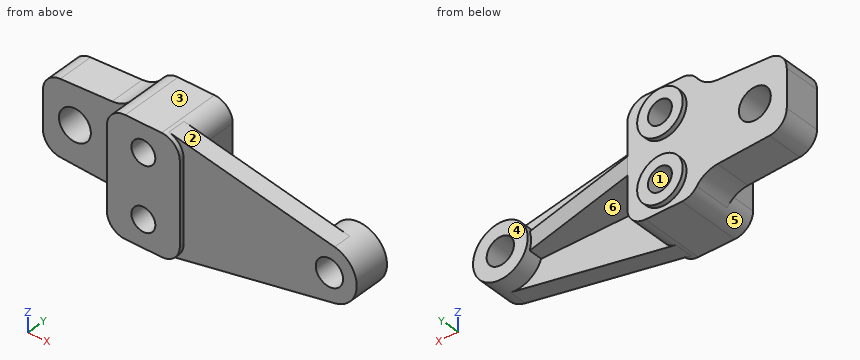
from build123d import *

# Parameters (mm, degrees)
SKETCH1_R                = 8.334375
SKETCH1_R_2              = 19.05
SKETCH1_R_3              = 9.525
SKETCH1_R_4              = 15.875
BOSS_EXTRUDE3_DEPTH      = 12.7
BOSS_EXTRUDE4_DEPTH      = 41.275
BOSS_EXTRUDE4_DEPTH_BACK = 3.175
SKETCH1_5_R              = 8.334375
SKETCH1_5_R_2            = 15.875
SKETCH1_6_R              = 19.05
SKETCH1_6_R_2            = 9.525
BOSS_EXTRUDE5_DEPTH      = 25.4
RIB1_START               = -6.35
RIB1_DEPTH               = 12.7
BOSS_EXTRUDE6_START      = 41.275
SKETCH1_7_R              = 15.875
SKETCH1_7_R_2            = 8.334375
BOSS_EXTRUDE6_DEPTH      = 3.175
BOSS_EXTRUDE8_START      = -25.4
SKETCH4_R                = 11.1125
BOSS_EXTRUDE8_DEPTH      = 25.4


# Read off the part's stored shape, not the designer's step: Rib1
with BuildPart() as part:
    # Sketch1 → Boss-Extrude3 (new body)
    # profile 1 of 5: a face of its own
    with BuildSketch(Plane(origin=(0, 0, 0), x_dir=(1, 0, 0), z_dir=(0, 1, 0))):
        with BuildLine():
            ThreePointArc((40.51167311, 41.043914661), (47.895872817, 36.657751744), (50.8, 28.575))
            Line((50.8, 28.575), (50.8, -28.575))
            ThreePointArc((50.8, -28.575), (47.895872817, -36.657751744), (40.51167311, -41.043914661))
            Line((40.51167311, -41.043914661), (156.017509664, -18.703371991))
            ThreePointArc((156.017509664, -18.703371991), (133.35, 0), (156.017509664, 18.703371991))
            Line((156.017509664, 18.703371991), (40.51167311, 41.043914661))
        make_face()
    # profile 2 of 5: a face of its own
    with BuildSketch(Plane(origin=(0, 0, 0), x_dir=(1, 0, 0), z_dir=(0, 1, 0))):
        with BuildLine():
            ThreePointArc((38.1, 41.275), (47.080256121, 37.555256121), (50.8, 28.575))
            Line((50.8, 28.575), (50.8, -28.575))
            ThreePointArc((50.8, -28.575), (47.080256121, -37.555256121), (38.1, -41.275))
            Line((38.1, -41.275), (12.7, -41.275))
            ThreePointArc((12.7, -41.275), (3.719743879, -37.555256121), (0, -28.575))
            Line((0, -28.575), (0, 28.575))
            ThreePointArc((0, 28.575), (3.719743879, 37.555256121), (12.7, 41.275))
            Line((12.7, 41.275), (38.1, 41.275))
        make_face()
        with Locations(Location((25.4, -22.225, 0), (0, 0, 270))):
            Circle(SKETCH1_R, mode=Mode.SUBTRACT)
        with Locations(Location((25.4, 22.225, 0), (0, 0, 270))):
            Circle(SKETCH1_R, mode=Mode.SUBTRACT)
    # profile 3 of 5: a face of its own
    with BuildSketch(Plane(origin=(0, 0, 0), x_dir=(1, 0, 0), z_dir=(0, 1, 0))):
        with Locations((152.4, 0)):
            Circle(SKETCH1_R_2)
        with Locations(Location((152.4, 0, 0), (0, 0, 270))):
            Circle(SKETCH1_R_3, mode=Mode.SUBTRACT)
    # profile 4 of 5: a face of its own
    with BuildSketch(Plane(origin=(0, 0, 0), x_dir=(1, 0, 0), z_dir=(0, 1, 0))):
        with Locations((25.4, 22.225)):
            Circle(SKETCH1_R_4)
        with Locations(Location((25.4, 22.225, 0), (0, 0, 270))):
            Circle(SKETCH1_R, mode=Mode.SUBTRACT)
    # profile 5 of 5: a face of its own
    with BuildSketch(Plane(origin=(0, 0, 0), x_dir=(1, 0, 0), z_dir=(0, 1, 0))):
        with Locations((25.4, -22.225)):
            Circle(SKETCH1_R_4)
        with Locations(Location((25.4, -22.225, 0), (0, 0, 270))):
            Circle(SKETCH1_R, mode=Mode.SUBTRACT)
    extrude(amount=BOSS_EXTRUDE3_DEPTH)

    # Sketch1<5> → Boss-Extrude4 (add, two sides: drawn at the far end of the back side and taken through both)
    # profile 1 of 3: a face of its own
    with BuildSketch(Plane(origin=(0, 0, 0), x_dir=(1, 0, 0), z_dir=(0, 1, 0)).offset(-BOSS_EXTRUDE4_DEPTH_BACK)):
        with BuildLine():
            ThreePointArc((38.1, 41.275), (47.080256121, 37.555256121), (50.8, 28.575))
            Line((50.8, 28.575), (50.8, -28.575))
            ThreePointArc((50.8, -28.575), (47.080256121, -37.555256121), (38.1, -41.275))
            Line((38.1, -41.275), (12.7, -41.275))
            ThreePointArc((12.7, -41.275), (3.719743879, -37.555256121), (0, -28.575))
            Line((0, -28.575), (0, 28.575))
            ThreePointArc((0, 28.575), (3.719743879, 37.555256121), (12.7, 41.275))
            Line((12.7, 41.275), (38.1, 41.275))
        make_face()
        with Locations(Location((25.4, -22.225, 0), (0, 0, 270))):
            Circle(SKETCH1_5_R, mode=Mode.SUBTRACT)
        with Locations(Location((25.4, 22.225, 0), (0, 0, 270))):
            Circle(SKETCH1_5_R, mode=Mode.SUBTRACT)
    # profile 2 of 3: a face of its own
    with BuildSketch(Plane(origin=(0, 0, 0), x_dir=(1, 0, 0), z_dir=(0, 1, 0)).offset(-BOSS_EXTRUDE4_DEPTH_BACK)):
        with Locations((25.4, -22.225)):
            Circle(SKETCH1_5_R_2)
        with Locations(Location((25.4, -22.225, 0), (0, 0, 270))):
            Circle(SKETCH1_5_R, mode=Mode.SUBTRACT)
    # profile 3 of 3: a face of its own
    with BuildSketch(Plane(origin=(0, 0, 0), x_dir=(1, 0, 0), z_dir=(0, 1, 0)).offset(-BOSS_EXTRUDE4_DEPTH_BACK)):
        with Locations((25.4, 22.225)):
            Circle(SKETCH1_5_R_2)
        with Locations(Location((25.4, 22.225, 0), (0, 0, 270))):
            Circle(SKETCH1_5_R, mode=Mode.SUBTRACT)
    extrude(amount=BOSS_EXTRUDE4_DEPTH + BOSS_EXTRUDE4_DEPTH_BACK)

    # Sketch1<6> → Boss-Extrude5 (add)
    with BuildSketch(Plane(origin=(0, 0, 0), x_dir=(1, 0, 0), z_dir=(0, 1, 0))):
        with Locations(Location((152.4, 0, 0), (0, 0, 79.053313044))):
            Circle(SKETCH1_6_R)
        with Locations(Location((152.4, 0, 0), (0, 0, 270))):
            Circle(SKETCH1_6_R_2, mode=Mode.SUBTRACT)
    extrude(amount=BOSS_EXTRUDE5_DEPTH)

    # Rib1 outline → Rib1 (add)
    with BuildSketch(Plane.XY.offset(RIB1_START)):
        Polygon((134.439487758, 22.361197239), (50.8, 41.275), (50.8, 12.7), (136, 12.7), (136, 22.008311042), align=None)
    extrude(amount=RIB1_DEPTH)

    # Sketch1<7> → Boss-Extrude6 (add)
    # profile 1 of 2: a face of its own
    with BuildSketch(Plane(origin=(0, 0, 0), x_dir=(1, 0, 0), z_dir=(0, 1, 0)).offset(BOSS_EXTRUDE6_START)):
        with Locations(Location((25.4, -22.225, 0), (0, 0, 270))):
            Circle(SKETCH1_7_R)
        with Locations(Location((25.4, -22.225, 0), (0, 0, 270))):
            Circle(SKETCH1_7_R_2, mode=Mode.SUBTRACT)
    # profile 2 of 2: a face of its own
    with BuildSketch(Plane(origin=(0, 0, 0), x_dir=(1, 0, 0), z_dir=(0, 1, 0)).offset(BOSS_EXTRUDE6_START)):
        with Locations(Location((25.4, 22.225, 0), (0, 0, 270))):
            Circle(SKETCH1_7_R)
        with Locations(Location((25.4, 22.225, 0), (0, 0, 270))):
            Circle(SKETCH1_7_R_2, mode=Mode.SUBTRACT)
    extrude(amount=BOSS_EXTRUDE6_DEPTH)

    # Sketch4 → Boss-Extrude8 (add)
    with BuildSketch(Plane(origin=(0, 41.275, 0), x_dir=(1, 0, 0), z_dir=(0, 1, 0)).offset(BOSS_EXTRUDE8_START)):
        with BuildLine():
            ThreePointArc((0, 28.575), (0.600462467, 32.43391066), (2.345069525, 35.927918798))
            ThreePointArc((2.345069525, 35.927918798), (-4.004870137, 30.266431204), (-12.186080417, 27.933627346))
            Line((-12.186080417, 27.933627346), (-48.292497181, 26.033289622))
            ThreePointArc((-48.292497181, 26.033289622), (-56.838230003, 22.091918232), (-60.325, 13.35084319))
            Line((-60.325, 13.35084319), (-60.325, -13.35084319))
            ThreePointArc((-60.325, -13.35084319), (-56.838230003, -22.091918232), (-48.292497181, -26.033289622))
            Line((-48.292497181, -26.033289622), (-12.186080417, -27.933627346))
            ThreePointArc((-12.186080417, -27.933627346), (-4.004870137, -30.266431204), (2.345069525, -35.927918798))
            ThreePointArc((2.345069525, -35.927918798), (0.600462467, -32.43391066), (0, -28.575))
            Line((0, -28.575), (0, 28.575))
        make_face()
        with Locations(Location((-38.1, 0, 0), (0, 0, 270))):
            Circle(SKETCH4_R, mode=Mode.SUBTRACT)
    extrude(amount=BOSS_EXTRUDE8_DEPTH)


solid = part.part
Design review of the part built by this model. Coordinates are the model's own, in mm. Face numbers are marked on the shaded views. A direction names the side the tool comes from. Give positions to 0.01 mm unless a question says otherwise; leave off trailing zeros. Order: outer loops, then holes, each group sorted by start corner. A loop starts at its lowest first (then second) coordinate and runs counter-clockwise, first axis right, second up. Notation, with made-up numbers: (-31.5, -7) - (7.5, -7) arc R15 ccw to (7.5, 13) - close; hole circle Ø6 at (-19, 23). An arc over 180 degrees is marked (long way). Write item = value, one per line. Start each with the question number.
Q1. We need section A-A on x = 25.4. State the section outline as (y, z) points (3 decimals).
Q2. Mouldability with a two-part tool opening along X and no side actions: class the marked faces 1, 2 and 3 as released by +X, released by -X, zero draft, split by the parting line, or undercut.
Q3. Clearance check with flat-ended pins moving along their axes: pin 1 Ø8 at (x, y) = (90.5, 29.5) entering from +Z; pin 2 Ø11 at (y, z) = (34, 20) entering from +X; pin 3 Ø11 at (y, z) = (27, -16) entering from +X; pin 4 Ø10 at (y, z) = (16, 16.5) entering from -X (3 decimals). State where each tip first meets the part, or that it passes through.
Q4. We need section B-B on y = 6. State how many separate pieces and enclosed holes the cut face has, plus the area to 3 significant figures.
Q5. We need section D-D on x = -38.1. State the section outline as (y, z) points (1 decimal).
Q6. To check wall thickness, follow L1, parallel to Z at x = 25, y = 17 (3 decimals); L2, parallel to X at y = 17.5, z = 17; L3, parallel to X at y = 19.5, z = 2 (3 decimals). State the ranges of each line that lie inside material, in increasing order. Write a range as from..to.
Q7. Tool access review of the marked faces 4, 5 and 6: name each direction out of +Z, -Z, +X, -X, +Y, -Y from which nothing blocks a thin tool from reaching the whole face with its end or side.
Working result:
q1.outline = (-3.175, -41.275) - (41.275, -41.275) - (41.275, -38.1) - (44.45, -38.1) - (44.45, -30.559) - (-3.175, -30.559) - close; (-3.175, -13.891) - (44.45, -13.891) - (44.45, -6.35) - (41.275, -6.35) - (41.275, 6.35) - (44.45, 6.35) - (44.45, 13.891) - (-3.175, 13.891) - close; (-3.175, 30.559) - (44.45, 30.559) - (44.45, 38.1) - (41.275, 38.1) - (41.275, 41.275) - (-3.175, 41.275) - close
q2.face_1 = undercut
q2.face_2 = released by +X
q2.face_3 = zero draft
q3.pin_1 = 6.35
q3.pin_2 = 50.8
q3.pin_3 = 168.14
q3.pin_4 = -60.325
q4.separate_pieces = 1
q4.enclosed_holes = 3
q4.area = 9,890 mm²
q5.outline = (15.9, -26.6) - (41.3, -26.6) - (41.3, -11.1) - (15.9, -11.1) - close; (15.9, 11.1) - (41.3, 11.1) - (41.3, 26.6) - (15.9, 26.6) - close
q6.L1 = -41.275..-30.55, -13.9..13.9, 30.55..41.275
q6.L2 = -59.79..18.91, 31.89..50.8, 143.8..161
q6.L3 = -60.325..-49.031, -27.169..143.087, 161.713..171.345
q7.face_4 = +Z, -Z, +X, +Y
q7.face_5 = -Z, -X, -Y
q7.face_6 = -Z, +Y
